Source: CAD feature listing. Evaluate the final solid. Frame: model axes, mm. A direction names the side the tool comes from. Give positions to 0.01 mm unless a question says otherwise; leave off trailing zeros. Order: outer loops, then holes, each group sorted by start corner. A loop starts at its lowest first (then second) coordinate and runs counter-clockwise, first axis right, second up. Notation, with made-up numbers: (19, 80) -> (33, 80) arc R29 ccw to (33, 106) -> close; hole circle Ø7 at (27, 89). An arc over 180 degrees is marked (long way). Use CSV: the item, a comma, the result in double quotes.
Autodesk Inventor part; units mm, degrees
ref_plane "Начальная плоскость" through (0, 0, -22.5) normal (0, 0, 1) x (1, 0, 0)
ref_plane "Конечная плоскость" through (0, 0, 2507.5) normal (0, 0, 1) x (1, 0, 0)
ref_plane "РабПлоскость4" through (-1.43, 0, -22.5) normal (0.7071, 0, -0.7071) x (-0.7071, 0, -0.7071)
ref_plane "Начальная плоскость" through (0, 0, -22.5) normal (0, 0, 1) x (1, 0, 0)
ref_plane "Конечная плоскость" through (0, 0, 2507.5) normal (0, 0, 1) x (1, 0, 0)
sketch "Эскиз" plane through (0, 0, 0) normal (0, 0, 1) x (1, 0, 0)
  line L0 (-1.43, 0) -> (-1.43, 40)
  line L1 (-1.43, 40) -> (43.57, 40)
  line L2 (43.57, 40) -> (43.57, 38.1774)
  line L3 (39.9881, 34.1993) -> (11.2338, 31.1771)
  line L4 (4.07, 23.221) -> (4.07, 0)
  line L5 (4.07, 0) -> (-1.43, 0) construction
  line L6 (23.82, 40) -> (23.82, 32.5) construction
  line L7 (43.57, 34.5758) -> (43.57, 32.5) construction
  line L8 (43.57, 32.5) -> (23.82, 32.5) construction
  line L9 (0, 15) -> (0, -27) construction
  line L10 (-5.539, 0) -> (16.0067, 0) construction
  line L11 (-1.43, 0) -> (-1.43, -40)
  line L12 (-1.43, -40) -> (43.57, -40)
  line L13 (43.57, -40) -> (43.57, -38.1774)
  line L14 (39.9881, -34.1993) -> (11.2338, -31.1771)
  line L15 (4.07, -23.221) -> (4.07, 0)
  arc A0 (11.2338, 31.1771) -> (4.07, 23.221) centre (12.07, 23.221) ccw
  arc A1 (4.07, -23.221) -> (11.2338, -31.1771) centre (12.07, -23.221) ccw
  arc A2 (39.9881, 34.1993) -> (43.57, 38.1774) centre (39.57, 38.1774) ccw
  arc A3 (43.57, -38.1774) -> (39.9881, -34.1993) centre (39.57, -38.1774) ccw
  line L16 (0, 56) -> (0, -56) construction
  line L17 (-15.5135, 0) -> (54.308, 0) construction
  point P0 (4.07, 30.4242)
  point P1 (43.57, -34.5758)
  point P2 (4.07, -30.4242)
  point P3 (23.82, -40)
  point P4 (23.82, -32.5)
  dimension "d0" = 5.5
  dimension "d1" = 40
  dimension "d2" = 45
  dimension "d3" = 7.5
  dimension "d4" = 19.75
  dimension "d5" = 2.0758
  dimension "d23" = 8
  dimension "d24" = 4
  dimension "d25" = 1.43
extrude "Тело" add sketch "Эскиз" along normal up to surface (2530 mm away) from surface at -22.5
sketch "Sketch3" plane through (0, 0, 0) normal (0, 0, 1) x (1, 0, 0)
  line L0 (0, 0) -> (10, 0)
ref_plane "Work Plane3" through (0, 0, 0) normal (0, -1, 0) x (1, 0, 0)
sketch "Sketch4" plane through (0, 0, 0) normal (0, -1, 0) x (1, 0, 0)
  line L0 (-2, -22.5) -> (12, -22.5)
  line L1 (-2, 2507.5) -> (12, 2507.5)
  dimension "d29" = 2530
ref_plane "РабПлоскость4" through (-1.43, 0, -22.5) normal (0.7071, 0, -0.7071) x (-0.7071, 0, -0.7071)
split "Разделение1" plane through (-1.43, 0, -22.5) removes the side toward (0.7071, 0, -0.7071)
ref_plane "РабПлоскость5" through (-1.43, 0, 2507.5) normal (0.7071, 0, 0.7071) x (0.7071, 0, -0.7071)
split "Разделение2" plane through (-1.43, 0, 2507.5) removes the side toward (0.7071, 0, 0.7071)
equation "\"d0\" = G_T"
equation "\"d1\" = 0.5 * G_H"
equation "\"d2\" = G_W"
equation "\"d3\" = G_T1"
equation "\"d4\" = G_C"
equation "\"d23\" = G_IR"
equation "\"d24\" = G_ER"
equation "\"d25\" = ex"
equation "\"d6\" = G_L"
equation "\"G_W\" = 45"
equation "\"G_T\" = 5.5"
equation "\"G_T1\" = 7.5"
equation "\"G_NG\" = 0.105104"
equation "\"G_ER\" = 4"
equation "\"G_IR\" = 8"
equation "\"G_C\" = 19.75"
equation "\"G_L\" = d29"
equation "\"ex\" = 1.43"
equation "\"G_OFFSET_START\" = 22.5"
equation "\"G_OFFSET_END\" = 22.5"
equation "\"d26\" = -G_OFFSET_START"
equation "\"d27\" = G_OFFSET_END + B_L"
equation "\"B_L\" = 2485"
properties part number "ISO 657/11 - CH 80 x 8 - 2530" material "Сталь нержавеющая, 440C"
1. Pin query (flat end, axial travel): P1, Ø23, axis at y = -4, z = 1220.5, coming from the +X side; P2, Ø6, axis at x = 17, y = -29.5, coming from the -Z side. Return the tip coordinate at first contact, or that it passes through.
Answer below:
P1,"stops at x = 4.07"
P2,"stops at z = -6.26"
2. Section query A-A on z = 1101.5. Return loops of the section in (x, y), plus the area to 3 significant figures.
Answer below:
outline,"(-1.43, -40) -> (43.57, -40) -> (43.57, -38.18) arc R4 ccw to (39.99, -34.2) -> (11.23, -31.18) arc R8 cw to (4.07, -23.22) -> (4.07, 23.22) arc R8 cw to (11.23, 31.18) -> (39.99, 34.2) arc R4 ccw to (43.57, 38.18) -> (43.57, 40) -> (-1.43, 40) -> close"
area,"1,050 mm²"
3. Section query B-B on x = 19.5. Return loops of the section in (y, z), plus the area to 3 significant figures.
Answer below:
outline,"(-40, -1.57) -> (-32.05, -1.57) -> (-32.05, 2486.57) -> (-40, 2486.57) -> close; (32.05, -1.57) -> (40, -1.57) -> (40, 2486.57) -> (32.05, 2486.57) -> close"
area,"39,600 mm²"
4. Section query C-C on y = 11. Return loops of the section in (x, z).
Answer below:
outline,"(-1.43, -22.5) -> (4.07, -17) -> (4.07, 2502) -> (-1.43, 2507.5) -> close"
5. Ray query, line 1 along Y through (x, z) = (36.5, 1053); line 2 along Y through (x, z) = (40, 895); line 3 along X through (y, z) = (19, 2187). Return the intervals inside material, ascending.
Answer below:
line 1,"y = -40 to -33.83, 33.83 to 40"
line 2,"y = -40 to -34.2, 34.2 to 40"
line 3,"x = -1.43 to 4.07"
6. Access query for faces 1 (the flat face through (4.07, 0, 1225)), 2 (the flat face through (-1.43, -1, 1225)). Directions: +Z, -Z, +X, -X, +Y, -Y. A direction counts if a zero-diameter tool reaches every point of the face in a straight line with its end or side. Return the directions, or none.
Answer below:
face 1,"+Z, -Z, +X"
face 2,"+Z, -Z, -X, +Y, -Y"
